Could you check a few things on this drawing? It's one solid part, dimensions in mm from its lowest x, y, z. Give positions to 0.01 mm unless a question says otherwise; leave off trailing zeros. Write each loop counter-clockwise with the first axis right and the second up, starting at its lowest first coordinate (ties: lowest second). Pieces come first, ordered by that corner, then holes. Notation, with made-up numbers: M -32,18 L 13,18 A20 ccw 13,48 Z; hole C 13,33.25 d6. An arc over 180 degrees is marked long. Write each question's results on one line, items separated by ' | '. Start each with the question number.
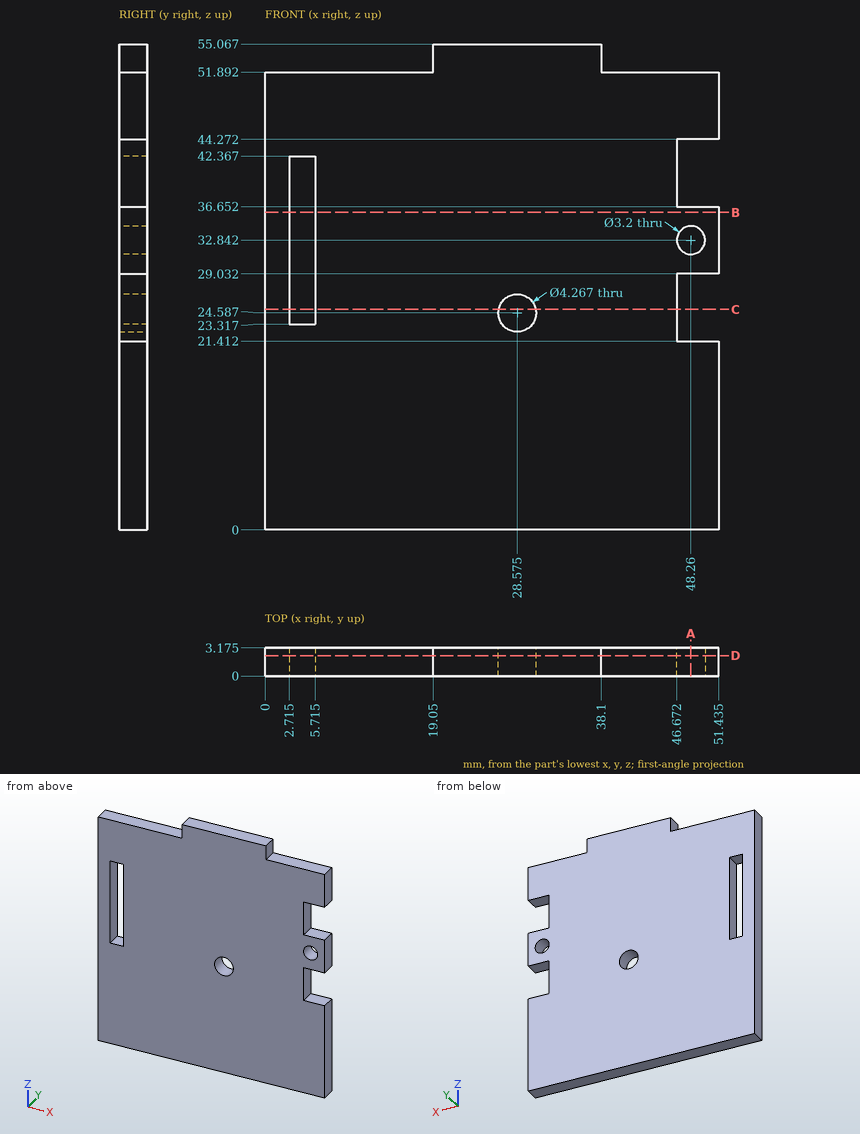
Q1. I'm going to push flat-ended pins straight in: P1, Ø1, axis at x = 48, y = 1.5, coming from the +Z side; P2, Ø1, axis at y = 2, z = 41, coming from the +X side; P3, Ø1, axis at y = 2.5, z = 52.5, coming from the +X side. Where does each tip first touch, or does it pass through?
Q2. If we section it at C-C (z = 25): Please give me the cut outline in (x, y) (1 decimal), plus the area to 3 significant figures.
Q3. If we section it at D-D (y = 2.3): Count the separate pieces of the cut face and the enclosed holes in it, plus the area to 3 significant figures.
Q4. Please list where these lines run through material, in increasing order: line 1 (Z direction, x = 48.26, y = 2.15); line 2 (X direction, y = 2.25, z = 26) (1 decimal); line 3 (Z direction, x = 49, y = 1.2) (1 decimal). Write a range as [from, to].
Q5. If we section it at B-B (z = 36): Please give me the cut outline in (x, y) (1 decimal), plus the area to 3 significant figures.
Q6. If we section it at A-A (x = 48.26): Please give me the cut outline in (y, z) (1 decimal), plus the area to 3 significant figures.
Determined:
1) P1: stops at z = 51.89 | P2: stops at x = 46.67 | P3: stops at x = 38.1
2) outline: M 0,0 L 2.7,0 L 2.7,3.2 L 0,3.2 Z; M 5.7,0 L 26.5,0 L 26.5,3.2 L 5.7,3.2 Z; M 30.7,0 L 46.7,0 L 46.7,3.2 L 30.7,3.2 Z | area: 125 mm²
3) separate pieces: 1 | enclosed holes: 3 | area: 2,580 mm²
4) line 1: z = [0, 21.41], [29.03, 31.24], [34.44, 36.65], [44.27, 51.89] | line 2: x = [0, 2.7], [5.7, 27], [30.2, 46.7] | line 3: z = [0, 21.4], [29, 31.4], [34.3, 36.7], [44.3, 51.9]
5) outline: M 0,0 L 2.7,0 L 2.7,3.2 L 0,3.2 Z; M 5.7,0 L 51.4,0 L 51.4,3.2 L 5.7,3.2 Z | area: 154 mm²
6) outline: M 0,0 L 3.2,0 L 3.2,21.4 L 0,21.4 Z; M 0,29 L 3.2,29 L 3.2,31.2 L 0,31.2 Z; M 0,34.4 L 3.2,34.4 L 3.2,36.7 L 0,36.7 Z; M 0,44.3 L 3.2,44.3 L 3.2,51.9 L 0,51.9 Z | area: 106 mm²
